Geometry: final body of the model. Coordinates: model frame, mm. Face numbers are marked on the shaded views. A direction names the side the tool comes from. Round coordinates to 2 decimals unless told otherwise and drop trailing zeros. Loops run counter-clockwise (first coordinate to the right, second up) from the corner with the lowest first, then second, coordinate; pieces in that order, holes last. Notation, with made-up numbers: (88.5, 24) - (136.5, 24) arc R13 cw to (136.5, 28) - close; hole circle Ø11 at (-38, -14). An arc over 180 degrees is marked (long way). Return JSON: item names as keys, results as strings. Group by question number.
1. Section A-A on x = 0. Return loops of the section in (y, z).
2. Section C-C on z = 10. Return loops of the section in (x, y).
3. Set-up query: the marked faces 1 and 2. Return all of +Z, -Z, +X, -X, +Y, -Y with unobstructed straight access to the full face (end or side cutting, diameter ignored); none if empty.
4. First-contact query: pin 1 Ø0.9 at (x, z) = (1.5, 0.5) entering from -Y; pin 2 Ø1 at (x, z) = (0, 18.5) entering from +Y; pin 3 Ø0.9 at (y, z) = (-1.5, 0) entering from +X. Flat tips, straight axial feed; report the tip coordinate or a pass-through.
5. Material intervals for probe 1 along Z at (x, y) = (0.35, 1.65); probe 2 along Z at (x, y) = (-1.3, 0.3); probe 3 along Y at (x, z) = (0.1, 20.25), sorted ascending.
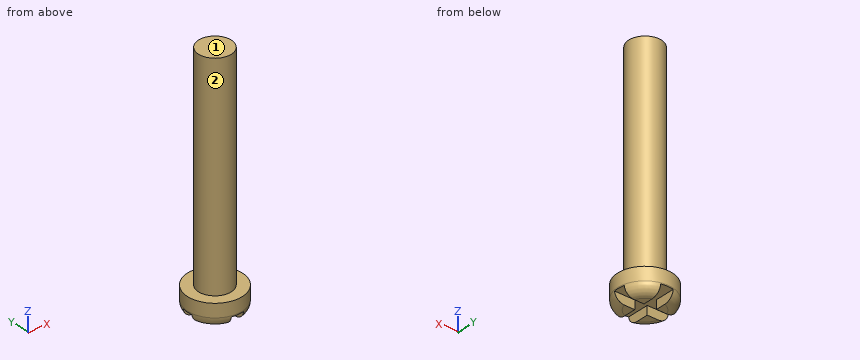
from build123d import *

# Parameters (mm, degrees)
F0_R     = 2.5
F1_DEPTH = 2.1
F2_R     = 1.5
F3_DEPTH = 19.6
F4_R     = 0.8932590181
F5_W     = 2.3426773259
F5_H     = 1.0091533186
F5_W_2   = 1.1473111808
F5_H_2   = 2.1985126659
F5_W_3   = 2.6310068788
F5_H_3   = 1.9702516729
F6_DEPTH = 0.8


with BuildPart() as f1:
    # F0 (on Top) → F1 (new body)
    with BuildSketch(Plane.XY):
        Circle(F0_R)
    extrude(amount=F1_DEPTH)

    # F2 (on face) → F3 (join)
    with BuildSketch(Plane.XY.offset(2.1)):
        Circle(F2_R)
    extrude(amount=F3_DEPTH)

    # F4
    f4_edges = [f1.edges().sort_by_distance(p)[0] for p in [
        (-2.5, 0, 0),
    ]]
    fillet(f4_edges, radius=F4_R)

    # F5 (on face) → F6 (cut)
    with BuildSketch(Plane(origin=(0, 0, 0), x_dir=(1, 0, 0), z_dir=(0, 0, -1))):
        with Locations((-1.7149599153, -0.0991132692)):
            Rectangle(F5_W, F5_H)
        with Locations((0.0300343381, 1.504719723)):
            Rectangle(F5_W_2, F5_H_2)
        with Locations((0.0300343381, -0.0991132692)):
            Rectangle(F5_W_2, F5_H)
        with Locations((1.9191933679, -0.0991132692)):
            Rectangle(F5_W_3, F5_H)
        with Locations((0.0300343381, -1.588815765)):
            Rectangle(F5_W_2, F5_H_3)
    extrude(amount=-F6_DEPTH, mode=Mode.SUBTRACT)


solid = f1.part
Taken from the geometry:
{
 "1": {"outline": "(-2.5, 0.8) - (2.5, 0.8) arc R0.89 ccw to (2.5, 0.89) - (2.5, 2.1) - (1.5, 2.1) - (1.5, 21.7) - (-1.5, 21.7) - (-1.5, 2.1) - (-2.5, 2.1) - (-2.5, 0.89) arc R0.89 ccw to start"},
 "2": {"outline": "circle Ø3 at (0, 0)"},
 "3": {"face 1": "+Z, +X, -X, +Y, -Y", "face 2": "+Z"},
 "4": {"pin 1": "y = -2.22", "pin 2": "y = 1.5", "pin 3": "x = 1.97"},
 "5": {"probe 1": "0.8 to 2.1", "probe 2": "0.8 to 21.7", "probe 3": "-1.5 to 1.5"}
}
